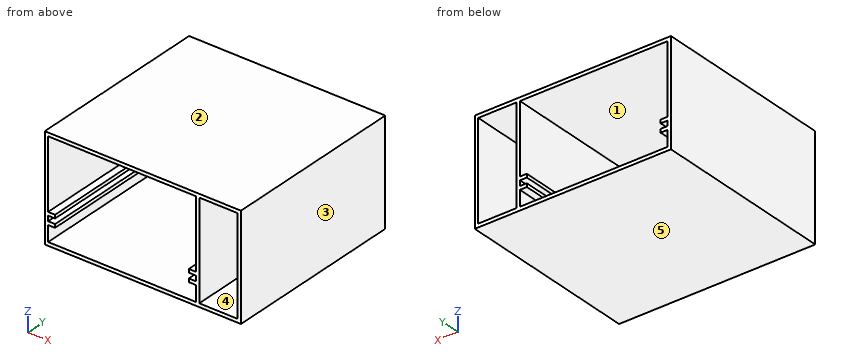
Autodesk Fusion 360 part; units mm, degrees
sketch "Esquisse1" plane through (0, 0, 0) normal (0, 1, 0) x (1, 0, 0)
  line L0 (0, 0) -> (-56.5, 0)
  line L1 (-56.5, 0) -> (-56.5, -30)
  line L2 (-56.5, -30) -> (0, -30)
  line L3 (0, -30) -> (0, 0)
  line L4 (-1, -29) -> (-55.5331, -29)
  line L5 (-55.5331, -29) -> (-55.5331, -1.0074)
  line L6 (-55.5331, -1.0074) -> (-1, -1.0074)
  line L7 (-1, -1.0074) -> (-1, -29)
  line L8 (-55.5331, -1.0074) -> (-1.0331, -1.0074)
  line L9 (-1.0331, -1.0074) -> (-1.0331, -28.0074)
  line L10 (-55.5331, -28.0074) -> (-55.5331, -1.0074)
  line L11 (-12, -29) -> (-13, -29)
  line L12 (-13, -29) -> (-13, -1)
  line L13 (-13, -1) -> (-12, -1)
  line L14 (-12, -1) -> (-12, -29)
  line L15 (-13, -9) -> (-15, -9)
  line L16 (-15, -9) -> (-15, -8)
  line L17 (-15, -8) -> (-13, -8)
  line L18 (-13, -8) -> (-13, -9)
  line L19 (-13, -6.485) -> (-15, -6.485)
  line L20 (-15, -6.485) -> (-15, -5.485)
  line L21 (-15, -5.485) -> (-13, -5.485)
  line L22 (-13, -5.485) -> (-13, -6.485)
  line L23 (-55.5331, -8.9771) -> (-53.5331, -8.9771)
  line L24 (-53.5331, -8.9771) -> (-53.5331, -7.9771)
  line L25 (-53.5331, -7.9771) -> (-55.5331, -7.9771)
  line L26 (-55.5331, -7.9771) -> (-55.5331, -8.9771)
  line L27 (-55.5331, -6.5064) -> (-53.5331, -6.5064)
  line L28 (-53.5331, -6.5064) -> (-53.5331, -5.5064)
  line L29 (-53.5331, -5.5064) -> (-55.5331, -5.5064)
  line L30 (-55.5331, -5.5064) -> (-55.5331, -6.5064)
extrude "Extrusion2" add sketch "Esquisse1" along normal blind 53 contours L0 L1 L2 L3 | L4 L6 L8 L11 L12 L14 L18 L22 | L12 L15 L16 L17 L18 | L12 L19 L20 L21 L22 | L5 L10 L23 L24 L25 L26 | L5 L10 L27 L28 L29 L30
sketch "Esquisse2" plane through (0, 0, 0) normal (0, -1, 0) x (1, 0, 0)
  line L0 (-12, 1.0074) -> (-12, 29)
  line L1 (-12, 29) -> (-1, 29)
  line L2 (-1, 29) -> (-1, 1.0074)
  line L3 (-1, 1.0074) -> (-12, 1.0074)
  line L4 (-12, 1.0074) -> (-12, 1)
  line L5 (-12, 1) -> (-13, 1)
  line L6 (-13, 1) -> (-13, 1.0074)
  line L7 (-13, 1.0074) -> (-55.5331, 1.0074)
  line L8 (-55.5331, 1.0074) -> (-55.5331, 5.5064)
  line L9 (-55.5331, 5.5064) -> (-53.5331, 5.5064)
  line L10 (-53.5331, 5.5064) -> (-53.5331, 6.5064)
  line L11 (-53.5331, 6.5064) -> (-55.5331, 6.5064)
  line L12 (-55.5331, 6.5064) -> (-55.5331, 7.9771)
  line L13 (-55.5331, 7.9771) -> (-53.5331, 7.9771)
  line L14 (-53.5331, 7.9771) -> (-53.5331, 8.9771)
  line L15 (-53.5331, 8.9771) -> (-55.5331, 8.9771)
  line L16 (-55.5331, 8.9771) -> (-55.5331, 29)
  line L17 (-55.5331, 29) -> (-13, 29)
  line L18 (-13, 29) -> (-13, 9)
  line L19 (-13, 9) -> (-15, 9)
  line L20 (-15, 9) -> (-15, 8)
  line L21 (-15, 8) -> (-13, 8)
  line L22 (-13, 8) -> (-13, 6.485)
  line L23 (-13, 6.485) -> (-15, 6.485)
  line L24 (-15, 6.485) -> (-15, 5.485)
  line L25 (-15, 5.485) -> (-13, 5.485)
  line L26 (-13, 5.485) -> (-13, 1.0074)
  line L27 (-13, 1.0074) -> (-12, 1.0074)
  line L28 (0, 0) -> (0, 30)
  line L29 (0, 30) -> (-56.5, 30)
  line L30 (-56.5, 30) -> (-56.5, 0)
  line L31 (-56.5, 0) -> (0, 0)
extrude "Extrusion1" [suppressed]
Model file for the job. Use its own axes, mm. Face numbers are marked on the shaded views. A direction names the side the tool comes from. Give positions to 0.01 mm unless a question says otherwise; leave off trailing zeros. Loops run counter-clockwise (first coordinate to the right, second up) from the corner with the lowest first, then second, coordinate; pieces in that order, holes last.
Item 1: Mould opens along X. For the marked faces 1, 2 and 3 say: +X half, -X half, draft (parallel to the pull), parting line (faces both ways), or undercut.
Check values:
face 1: undercut
face 2: draft
face 3: +X half
Item 2: Slice it at A-A (x = -28). Write the cut outline in (y, z).
Check values:
outline: (0, 0) - (53, 0) - (53, 1.01) - (0, 1.01) - close; (0, 29) - (53, 29) - (53, 30) - (0, 30) - close
Item 3: Drill centre lines: line 1 along X through (y, z) = (6.5, 8.75); line 2 along X through (y, z) = (6.5, 3.5); line 3 along Z through (x, y) = (-51, 16). Where is each one in solid material? Low to high.
Check values:
line 1: x = -56.5 to -53.53, -15 to -12, -1 to 0
line 2: x = -56.5 to -55.53, -13 to -12, -1 to 0
line 3: z = 0 to 1.01, 29 to 30
Item 4: Slice it at B-B (z = 28.25). Write the cut outline in (x, y).
Check values:
outline: (-56.5, 0) - (-55.53, 0) - (-55.53, 53) - (-56.5, 53) - close; (-13, 0) - (-12, 0) - (-12, 53) - (-13, 53) - close; (-1, 0) - (0, 0) - (0, 53) - (-1, 53) - close
Item 5: Which spindle directions (+Z, -Z, +X, -X, +Y, -Y) get a long thin tool onto all of the face, cutting with end or side? Do the marked faces 4 and 5. Say none if no direction does.
Check values:
face 4: +Y, -Y
face 5: -Z, +X, -X, +Y, -Y
